Build history of the part. All positions in model axes, mm. Face numbers are marked on the shaded views. Coordinates: 2 decimals unless noted, no trailing zeros. Order: outer loops, then holes, each group sorted by start corner. A loop starts at its lowest first (then second) coordinate and runs counter-clockwise, first axis right, second up. Notation, with made-up numbers: (-3, 70.5) - (19, 70.5) arc R20 ccw to (19, 92.5) - close; hole circle Ø3 at (20.25, -28.75). An arc over 180 degrees is marked (long way). Write each question's results on one line, items separated by ' | '. Start each with the question number.
from build123d import *

# Parameters (mm, degrees)
DODANIE_WYCI_GNI_CIE1_DEPTH = 5
SZKIC2_R                    = 5
WYTNIJ_WYCI_GNI_CIE1_DEPTH  = 5
SFAZOWANIE1_SIZE            = 0.5
SZKIC6_OUTSIDE_W            = 56.99
SZKIC6_OUTSIDE_H            = 54.846
SZKIC6_OUTSIDE_R            = 6.92820323
WYTNIJ_WYCI_GNI_CIE2_DEPTH  = 10
WYTNIJ_WYCI_GNI_CIE2_DRAFT  = -60
SZKIC7_OUTSIDE_W            = 56.99
SZKIC7_OUTSIDE_H            = 54.846
SZKIC7_OUTSIDE_R            = 6.92820323
WYTNIJ_WYCI_GNI_CIE3_DEPTH  = 10
WYTNIJ_WYCI_GNI_CIE3_DRAFT  = -60


with BuildPart() as part:
    # Szkic1 → Dodanie-wyciągnięcie1 (new body)
    with BuildSketch(Plane.XY):
        Polygon((-4, 6.92820323), (-8, 0), (-4, -6.92820323), (4, -6.92820323), (8, 0), (4, 6.92820323), align=None)
    extrude(amount=DODANIE_WYCI_GNI_CIE1_DEPTH)

    # Szkic2 → Wytnij-wyciągnięcie1 (cut)
    with BuildSketch(Plane.XY.offset(5)):
        Circle(SZKIC2_R)
    extrude(amount=-WYTNIJ_WYCI_GNI_CIE1_DEPTH, mode=Mode.SUBTRACT)

    # Sfazowanie1
    sfazowanie1_edges = [part.edges().sort_by_distance(p)[0] for p in [
        (-5, 0, 0),
        (-5, 0, 5),
    ]]
    chamfer(sfazowanie1_edges, length=SFAZOWANIE1_SIZE)


with BuildPart() as wytnij_wyci_gni_cie2_tool:
    # Szkic6 outside → Wytnij-wyciągnięcie2 (with draft: the straight prism first)
    with BuildSketch(Plane(origin=(0, 0, 0), x_dir=(-1, 0, 0), z_dir=(0, 0, -1))):
        Rectangle(SZKIC6_OUTSIDE_W, SZKIC6_OUTSIDE_H)
        Circle(SZKIC6_OUTSIDE_R, mode=Mode.SUBTRACT)
    extrude(amount=-WYTNIJ_WYCI_GNI_CIE2_DEPTH)
    # Wytnij-wyciągnięcie2: the draft: its side faces are tilted about the plane it starts from
    wytnij_wyci_gni_cie2_sides = [wytnij_wyci_gni_cie2_tool.faces().sort_by_distance(p)[0] for p in [
        (0, -27.423, 5),
        (-28.495, 0, 5),
        (0, 27.423, 5),
        (28.495, 0, 5),
        (6.92820323, 0, 5),
    ]]
    draft(wytnij_wyci_gni_cie2_sides, Plane(origin=(0, 0, 0), x_dir=(-1, 0, 0), z_dir=(0, 0, -1)), WYTNIJ_WYCI_GNI_CIE2_DRAFT)


with BuildPart() as part_1:
    add(part.part)

    # Wytnij-wyciągnięcie2: cut by wytnij_wyci_gni_cie2_tool
    add(wytnij_wyci_gni_cie2_tool.part, mode=Mode.SUBTRACT)


with BuildPart() as wytnij_wyci_gni_cie3_tool:
    # Szkic7 outside → Wytnij-wyciągnięcie3 (with draft: the straight prism first)
    with BuildSketch(Plane.XY.offset(5)):
        Rectangle(SZKIC7_OUTSIDE_W, SZKIC7_OUTSIDE_H)
        Circle(SZKIC7_OUTSIDE_R, mode=Mode.SUBTRACT)
    extrude(amount=-WYTNIJ_WYCI_GNI_CIE3_DEPTH)
    # Wytnij-wyciągnięcie3: the draft: its side faces are tilted about the plane it starts from
    wytnij_wyci_gni_cie3_sides = [wytnij_wyci_gni_cie3_tool.faces().sort_by_distance(p)[0] for p in [
        (0, -27.423, 0),
        (28.495, 0, 0),
        (0, 27.423, 0),
        (-28.495, 0, 0),
        (-6.92820323, 0, 0),
    ]]
    draft(wytnij_wyci_gni_cie3_sides, Plane.XY.offset(5), WYTNIJ_WYCI_GNI_CIE3_DRAFT)


with BuildPart() as part_2:
    add(part_1.part)

    # Wytnij-wyciągnięcie3: cut by wytnij_wyci_gni_cie3_tool
    add(wytnij_wyci_gni_cie3_tool.part, mode=Mode.SUBTRACT)


solid = part_2.part
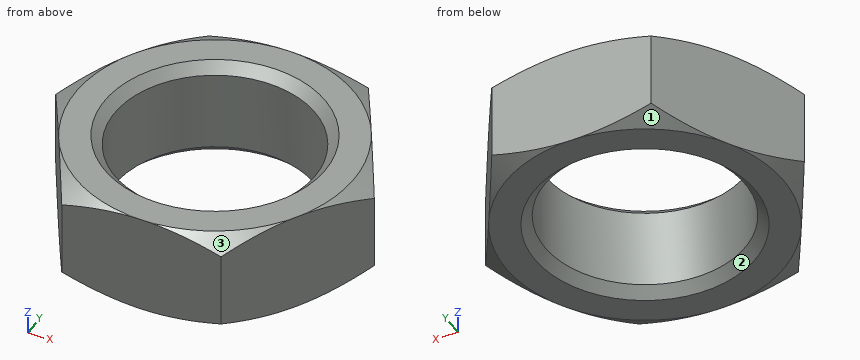
Item 1: Flat gauge pins, fed straight in: P1, Ø1.5, axis at y = -3.5, z = 2, coming from the -X side; P2, Ø3, axis at y = -2, z = 2.5, coming from the -X side. Where does each tip first touch, or does it go through?
Item 2: Slice it at A-A (z = 1). Write the cut outline in (x, y).
Item 3: Pull direction X, two halves, no side cores. Call the marked faces 1, 2 and 3: released by +X, released by -X, zero draft, split by the parting line, or undercut.
Item 4: Probe probe 1 along Y at (x, z) = (0, 2.9); probe 2 along Y at (x, z) = (3, 1.85); probe 3 along X at (y, z) = (1.5, 0.75). List the from-to ranges inside material, lowest first.
Resolved:
1) P1: x = -6.41 | P2: x = -7.71
2) outline: (-8, 0) - (-4, -6.93) - (4, -6.93) - (8, 0) - (4, 6.93) - (-4, 6.93) - close; hole circle Ø10 at (0, 0)
3) face 1: released by -X | face 2: undercut | face 3: released by +X
4) probe 1: -6.93 to -5, 5 to 6.93 | probe 2: -6.93 to -4, 4 to 6.93 | probe 3: -7.13 to -4.77, 4.77 to 7.13
